from build123d import *

# Parameters (mm, degrees)
SKETCH1_W           = 76.2
SKETCH1_H           = 36.83
SKETCH1_R           = 1.0999978
SKETCH1_R_2         = 2.159
BOSS_EXTRUDE1_DEPTH = 38.1
SKETCH3_R           = 2.54
CUT_EXTRUDE2_DEPTH  = 36.83
SKETCH4_W           = 19.685
SKETCH4_H           = 36.83
CUT_EXTRUDE3_DEPTH  = 35.56
CUT_EXTRUDE4_DEPTH  = 35.56


with BuildPart() as part:
    # Sketch1 → Boss-Extrude1 (new body)
    with BuildSketch(Plane(origin=(0, 0, 0), x_dir=(1, 0, 0), z_dir=(0, 1, 0))):
        with Locations((-1.422532637, -3.27613577)):
            Rectangle(SKETCH1_W, SKETCH1_H)
        with Locations(Location((-16.422528037, 11.72385963, 0), (0, 0, 90))):
            Circle(SKETCH1_R, mode=Mode.SUBTRACT)
        with Locations(Location((13.577462763, 11.72385963, 0), (0, 0, 90))):
            Circle(SKETCH1_R, mode=Mode.SUBTRACT)
        with Locations(Location((13.577462763, -18.27613117, 0), (0, 0, 90))):
            Circle(SKETCH1_R, mode=Mode.SUBTRACT)
        with Locations(Location((-16.422528037, -18.27613117, 0), (0, 0, 90))):
            Circle(SKETCH1_R, mode=Mode.SUBTRACT)
        with Locations(Location((31.597467363, -15.34113577, 0), (0, 0, 90))):
            Circle(SKETCH1_R_2, mode=Mode.SUBTRACT)
        with Locations(Location((31.597467363, 8.78886423, 0), (0, 0, 90))):
            Circle(SKETCH1_R_2, mode=Mode.SUBTRACT)
        with Locations(Location((-34.442532637, -15.34113577, 0), (0, 0, 90))):
            Circle(SKETCH1_R_2, mode=Mode.SUBTRACT)
        with Locations(Location((-34.442532637, 8.78886423, 0), (0, 0, 90))):
            Circle(SKETCH1_R_2, mode=Mode.SUBTRACT)
    extrude(amount=BOSS_EXTRUDE1_DEPTH)

    # Sketch3 → Cut-Extrude2 (cut)
    with BuildSketch(Plane.XZ):
        with Locations(Location((-16.422528037, 18.27613117, 0), (0, 0, 270))):
            Circle(SKETCH3_R)
        with Locations(Location((13.577462763, 18.27613117, 0), (0, 0, 90))):
            Circle(SKETCH3_R)
        with Locations(Location((13.577462763, -11.72385963, 0), (0, 0, 270))):
            Circle(SKETCH3_R)
        with Locations(Location((-16.422528037, -11.72385963, 0), (0, 0, 90))):
            Circle(SKETCH3_R)
    extrude(amount=-CUT_EXTRUDE2_DEPTH, mode=Mode.SUBTRACT)

    # Sketch4 → Cut-Extrude3 (cut)
    with BuildSketch(Plane(origin=(0, 38.1, 0), x_dir=(1, 0, 0), z_dir=(0, 1, 0))):
        with Locations((-29.680032637, -3.27613577)):
            Rectangle(SKETCH4_W, SKETCH4_H)
        with Locations((26.834967363, -3.27613577)):
            Rectangle(SKETCH4_W, SKETCH4_H)
    extrude(amount=-CUT_EXTRUDE3_DEPTH, mode=Mode.SUBTRACT)

    # Sketch5 → Cut-Extrude4 (cut)
    with BuildSketch(Plane.XZ):
        Polygon((9.767462763, -7.91385963), (9.767462763, -11.72385963), (-12.612528037, -11.72385963), (-12.612528037, -7.91385963), (-16.422528037, -7.91385963), (-16.422528037, 14.46613117), (-12.612528037, 14.46613117), (-12.612528037, 18.27613117), (9.767462763, 18.27613117), (9.767462763, 14.46613117), (13.577462763, 14.46613117), (13.577462763, -7.91385963), align=None)
    extrude(amount=-CUT_EXTRUDE4_DEPTH, mode=Mode.SUBTRACT)


solid = part.part
Geometry check sheet. Reference: the model listing, model coordinates, mm. A direction names the side the tool comes from. Coordinates: 2 decimals unless noted, no trailing zeros. Loops run counter-clockwise (first coordinate to the right, second up) from the corner with the lowest first, then second, coordinate; pieces in that order, holes last. Notation, with made-up numbers: (79.5, -21.5) - (113.5, -21.5) arc R25 cw to (113.5, -5.5) - close; hole circle Ø6 at (54, 14). An arc over 180 degrees is marked (long way). Use one line per item in the form item = value. Start each with the question number.
Item 1: Gauge pin test, flat ends, axial feed: pin 1 (4 mm diameter, centred on y = 15, z = -10, fed in from -X); pin 2 (3 mm diameter, centred on y = 13.5, z = 15.5, fed in from +X); pin 3 (4.5 mm diameter, centred on x = -16.42, z = -11.72, fed in from -Y). Record the tip position at first contact, or that the pin passes through.
Item 2: Section check A-A, the plane y = 29. Enter the section's corners in (x, z).
Item 3: Section check B-B, the plane z = 11. Enter the section's corners in (x, y), and give its area (3 significant figures).
Item 4: Mould release check, pull along X, two halves, no side actions. Record for faces 1 (the face through (-2, 38.1, 3)), 2 (the face through (16.992, 21, 4)), 3 (the face through (12.834, 37.456, -10.913)): +X half, -X half, draft (parallel to the pull), parting line (faces both ways), or undercut.
Item 5: Section check C-C, the plane x = -7. Enter the section's corners in (y, z), and give its area (3 significant figures).
Item 6: Tool access check on faces 4 (the face through (36.677, 1, 4)), 5 (the face through (-15, 18, 14.466)). Record the directions out of +Z, -Z, +X, -X, +Y, -Y that give a thin tool (end or side, any length) a straight path to the whole face; none if there is none.
Item 7: Section check D-D, the plane x = 24. Enter the section's corners in (y, z).
Item 8: Thickness scan on probe 1 along X at (y, z) = (34, -6); probe 2 along X at (y, z) = (27.5, -9); probe 3 along X at (y, z) = (35.5, -10). Record the ranges inside material, lowest first.
Computed:
q1.pin_1 = -19.84
q1.pin_2 = 16.99
q1.pin_3 = 36.83
q2.outline = (-19.84, -15.14) - (16.99, -15.14) - (16.99, 21.69) - (-19.84, 21.69) - close; hole circle Ø5.08 at (-16.42, -11.72); hole circle Ø5.08 at (-16.42, 18.28); hole (-16.42, -7.91) - (-12.61, -7.91) - (-12.61, -11.72) - (9.77, -11.72) - (9.77, -7.91) - (13.58, -7.91) - (13.58, 14.47) - (9.77, 14.47) - (9.77, 18.28) - (-12.61, 18.28) - (-12.61, 14.47) - (-16.42, 14.47) - close; hole circle Ø5.08 at (13.58, -11.72); hole circle Ø5.08 at (13.58, 18.28)
q3.outline = (-39.52, 0) - (-16.42, 0) - (-16.42, 35.56) - (13.58, 35.56) - (13.58, 0) - (36.68, 0) - (36.68, 2.54) - (16.99, 2.54) - (16.99, 38.1) - (-19.84, 38.1) - (-19.84, 2.54) - (-39.52, 2.54) - close
q3.area = 436 mm2
q4.face_1 = draft
q4.face_2 = +X half
q4.face_3 = undercut
q5.outline = (0, -15.14) - (38.1, -15.14) - (38.1, 21.69) - (0, 21.69) - (0, 18.28) - (35.56, 18.28) - (35.56, -11.72) - (0, -11.72) - close
q5.area = 336 mm2
q6.face_4 = +Z, -Z, +X, +Y, -Y
q6.face_5 = -Y
q7.outline = (0, -15.14) - (2.54, -15.14) - (2.54, 21.69) - (0, 21.69) - close
q8.probe_1 = -19.84 to -16.42, 13.58 to 16.99
q8.probe_2 = -19.84 to -12.61, 9.77 to 16.99
q8.probe_3 = -19.84 to -18.29, -14.56 to -12.61, 9.77 to 11.71, 15.44 to 16.99
